Work out the finished part from the listing and answer in its coordinate system (mm). A direction names the side the tool comes from. Give positions to 0.01 mm unless a question says otherwise; leave off trailing zeros. Loops run counter-clockwise (first coordinate to the right, second up) from the corner with the lowest first, then second, coordinate; pieces in that order, holes last.
```python
from build123d import *

# Parameters (mm, degrees)
SKETCH_W        = 116.73
SKETCH_H        = 71.06
PAD_DEPTH       = 30
THICKNESS_T     = -3
SKETCH001_W     = 10.600402
SKETCH001_H     = 12.306634
SKETCH001_W_2   = 9.956932
SKETCH001_H_2   = 8.02499
SKETCH001_W_3   = 10.164987
SKETCH001_H_3   = 7.995267
POCKET_DEPTH    = 5
SKETCH005_R     = 1.5
SKETCH005_R_2   = 0.75
PAD004_DEPTH    = 26
PAD005_DEPTH    = 26
PAD006_DEPTH    = 26
PAD007_DEPTH    = 26
SKETCH004_W     = 43.838747
SKETCH004_H     = 11.498687
POCKET001_DEPTH = 5
FILLET_R        = 4
FILLET002_R     = 4
FILLET003_R     = 4
FILLET004_R     = 1
FILLET005_R     = 1
FILLET006_R     = 1


with BuildPart() as part:
    # Sketch → Pad (new body)
    with BuildSketch(Plane.XY):
        with Locations((54.802781, 32.357444)):
            Rectangle(SKETCH_W, SKETCH_H)
    extrude(amount=PAD_DEPTH)

    # Thickness
    thickness_openings = [part.faces().sort_by_distance(p)[0] for p in [
        (54.802781, 32.357444, 30),
    ]]
    offset(amount=THICKNESS_T, openings=thickness_openings, kind=Kind.INTERSECTION)

    # Sketch001 (on Face3 of Thickness) → Pocket (cut)
    with BuildSketch(Plane.YZ.offset(113.167781)):
        with Locations((53.013897, 10.526186)):
            Rectangle(SKETCH001_W, SKETCH001_H)
        with Locations((13.300911, 8.478813)):
            Rectangle(SKETCH001_W_2, SKETCH001_H_2)
        with Locations((25.531591, 8.493675)):
            Rectangle(SKETCH001_W_3, SKETCH001_H_3)
    extrude(amount=-POCKET_DEPTH, mode=Mode.SUBTRACT)

    # Sketch005 (on Face23 of Pocket) → Pad004 (join)
    with BuildSketch(Plane.XY.offset(3)):
        with Locations((3.543065, 60.674728)):
            Circle(SKETCH005_R)
        with Locations((3.543065, 60.674728)):
            Circle(SKETCH005_R_2, mode=Mode.SUBTRACT)
        with Locations((106.043365, 60.956181)):
            Circle(SKETCH005_R)
        with Locations((106.043365, 60.956181)):
            Circle(SKETCH005_R_2, mode=Mode.SUBTRACT)
        with Locations((3.308966, 3.559068)):
            Circle(SKETCH005_R)
        with Locations((3.308966, 3.559068)):
            Circle(SKETCH005_R_2, mode=Mode.SUBTRACT)
        with Locations((106.180908, 3.540333)):
            Circle(SKETCH005_R)
        with Locations((106.180908, 3.540333)):
            Circle(SKETCH005_R_2, mode=Mode.SUBTRACT)
    extrude(amount=PAD004_DEPTH)

    # Sketch005 (on Face23 of Pocket) → Pad005 (join)
    with BuildSketch(Plane.XY.offset(3)):
        with Locations((3.543065, 60.674728)):
            Circle(SKETCH005_R)
        with Locations((3.543065, 60.674728)):
            Circle(SKETCH005_R_2, mode=Mode.SUBTRACT)
        with Locations((106.043365, 60.956181)):
            Circle(SKETCH005_R)
        with Locations((106.043365, 60.956181)):
            Circle(SKETCH005_R_2, mode=Mode.SUBTRACT)
        with Locations((3.308966, 3.559068)):
            Circle(SKETCH005_R)
        with Locations((3.308966, 3.559068)):
            Circle(SKETCH005_R_2, mode=Mode.SUBTRACT)
        with Locations((106.180908, 3.540333)):
            Circle(SKETCH005_R)
        with Locations((106.180908, 3.540333)):
            Circle(SKETCH005_R_2, mode=Mode.SUBTRACT)
    extrude(amount=PAD005_DEPTH)

    # Sketch005 (on Face23 of Pocket) → Pad006 (join)
    with BuildSketch(Plane.XY.offset(3)):
        with Locations((3.543065, 60.674728)):
            Circle(SKETCH005_R)
        with Locations((3.543065, 60.674728)):
            Circle(SKETCH005_R_2, mode=Mode.SUBTRACT)
        with Locations((106.043365, 60.956181)):
            Circle(SKETCH005_R)
        with Locations((106.043365, 60.956181)):
            Circle(SKETCH005_R_2, mode=Mode.SUBTRACT)
        with Locations((3.308966, 3.559068)):
            Circle(SKETCH005_R)
        with Locations((3.308966, 3.559068)):
            Circle(SKETCH005_R_2, mode=Mode.SUBTRACT)
        with Locations((106.180908, 3.540333)):
            Circle(SKETCH005_R)
        with Locations((106.180908, 3.540333)):
            Circle(SKETCH005_R_2, mode=Mode.SUBTRACT)
    extrude(amount=PAD006_DEPTH)

    # Sketch005 (on Face23 of Pocket) → Pad007 (join)
    with BuildSketch(Plane.XY.offset(3)):
        with Locations((3.543065, 60.674728)):
            Circle(SKETCH005_R)
        with Locations((3.543065, 60.674728)):
            Circle(SKETCH005_R_2, mode=Mode.SUBTRACT)
        with Locations((106.043365, 60.956181)):
            Circle(SKETCH005_R)
        with Locations((106.043365, 60.956181)):
            Circle(SKETCH005_R_2, mode=Mode.SUBTRACT)
        with Locations((3.308966, 3.559068)):
            Circle(SKETCH005_R)
        with Locations((3.308966, 3.559068)):
            Circle(SKETCH005_R_2, mode=Mode.SUBTRACT)
        with Locations((106.180908, 3.540333)):
            Circle(SKETCH005_R)
        with Locations((106.180908, 3.540333)):
            Circle(SKETCH005_R_2, mode=Mode.SUBTRACT)
    extrude(amount=PAD007_DEPTH)

    # Sketch004 → Pocket001 (cut)
    with BuildSketch(Plane(origin=(-3.562219, 0, 0), x_dir=(0, -1, 0), z_dir=(-1, 0, 0))):
        with Locations((-38.438376, 21.701757)):
            Rectangle(SKETCH004_W, SKETCH004_H)
    extrude(amount=-POCKET001_DEPTH, mode=Mode.SUBTRACT)

    # Fillet
    fillet_edges = [part.edges().sort_by_distance(p)[0] for p in [
        (-3.562219, -3.172556, 15),
    ]]
    fillet(fillet_edges, radius=FILLET_R)

    # Fillet002
    fillet002_edges = [part.edges().sort_by_distance(p)[0] for p in [
        (-3.562219, 67.887444, 15),
        (113.167781, 67.887444, 15),
    ]]
    fillet(fillet002_edges, radius=FILLET002_R)

    # Fillet003
    fillet003_edges = [part.edges().sort_by_distance(p)[0] for p in [
        (113.167781, -3.172556, 15),
    ]]
    fillet(fillet003_edges, radius=FILLET003_R)

    # Fillet004
    fillet004_edges = [part.edges().sort_by_distance(p)[0] for p in [
        (-0.562219, 64.887444, 16.5),
    ]]
    fillet(fillet004_edges, radius=FILLET004_R)

    # Fillet005
    fillet005_edges = [part.edges().sort_by_distance(p)[0] for p in [
        (110.167781, 64.887444, 16.5),
    ]]
    fillet(fillet005_edges, radius=FILLET005_R)

    # Fillet006
    fillet006_edges = [part.edges().sort_by_distance(p)[0] for p in [
        (110.167781, -0.172556, 16.5),
        (-0.562219, -0.172556, 16.5),
    ]]
    fillet(fillet006_edges, radius=FILLET006_R)


with BuildPart() as part_1:
    # Body placement: moved
    add(part.part.moved(Location((0, 0, -5))))


solid = part_1.part
```
Q1. Section C-C on y = 23.5 is taken. Give the vertices of the cut face in (x, z), plus the area to 3 significant figures.
Q2. Section B-B on z = 16.5 is taken. State how many separate pieces and enclosed holes the cut face has, plus the area to 3 significant figures.
Q3. Section D-D on x = 103 is taken. Give the vertices of the cut face in (y, z).
Q4. Determine the mould class of faces 1 (the face through (54, 67.887, 10)), 2 (the face through (112, 58.314, 5)), 3 (the face through (54, 33, -2)) for opening direction Z: +Z half, -Z half, draft (parallel to the pull), parting line (faces both ways), or undercut.
Q5. Consider line 1 along Y through (x, z) = (2, 5); line 2 along Y through (x, z) = (26.5, 2); line 3 along X through (y, z) = (2, 1.25). Determine where each line is inside the solid, lowest interval first.
Q6. Given pin 1 (1.5 mm diameter, centred on x = 112, z = 2.5, fed in from -Y); pin 2 (1.5 mm diameter, centred on x = 111, z = 8.5, fed in from +Y); pin 3 (10 mm diameter, centred on x = 44, y = 28.5, fed in from +Z), each flat-ended and moving along its own axis, determine where each tip first touches the part or whether it passes through.
Q7. Which of the six approach directions +Z, -Z, +X, -X, +Y, -Y give full straight-line access (tool end or side, diameter ignored) to faces 4 (the face through (107.61, 3.99, 10.82)), 5 (the face through (50, -2, 25)), 6 (the face through (112, 18.279, 3)), 7 (the face through (-2, 39, 22.451)), 8 (the face through (54, 33, -5))?
Q8. Section A-A on y = 12.5 is taken. Give the vertices of the cut face in (x, z), plus the area to 3 significant figures.
Check result:
1. outline: (-3.56, -5) - (113.17, -5) - (113.17, -0.5) - (110.17, -0.5) - (110.17, -2) - (-0.56, -2) - (-0.56, 10.95) - (-3.56, 10.95) - close; (-3.56, 22.45) - (-0.56, 22.45) - (-0.56, 25) - (-3.56, 25) - close; (110.17, 7.49) - (113.17, 7.49) - (113.17, 25) - (110.17, 25) - close
1. area: 454 mm2
2. separate pieces: 5
2. enclosed holes: 4
2. area: 968 mm2
3. outline: (-3.17, -5) - (67.89, -5) - (67.89, 25) - (64.89, 25) - (64.89, -2) - (-0.17, -2) - (-0.17, 25) - (-3.17, 25) - close
4. face 1: draft
4. face 2: undercut
4. face 3: +Z half
5. line 1: y = -3.17 to -0.17, 2.83 to 4.29, 64.89 to 67.89
5. line 2: y = -3.17 to -0.17, 64.89 to 67.89
5. line 3: x = -3.56 to -0.56, 110.17 to 113.17
6. pin 1: stops at y = -2.59
6. pin 2: stops at y = 67.74
6. pin 3: stops at z = -2
7. face 4: +Z
7. face 5: +Z, +X, -X, +Y, -Y
7. face 6: +X
7. face 7: -X
7. face 8: -Z, +X, -X, +Y, -Y
8. outline: (-3.56, -5) - (113.17, -5) - (113.17, -0.53) - (110.17, -0.53) - (110.17, -2) - (-0.56, -2) - (-0.56, 25) - (-3.56, 25) - close; (110.17, 7.49) - (113.17, 7.49) - (113.17, 25) - (110.17, 25) - close
8. area: 488 mm2
